Build history of the part. All positions in model axes, mm. A direction names the side the tool comes from. Round coordinates to 2 decimals unless told otherwise and drop trailing zeros. One line per question, with ' | ' between items.
Autodesk Inventor part; units mm, degrees
ref_plane "Work Plane1" through (-1.711, 0.0003, 0) normal (0, 1, 0) x (1, 0, 0)
ref_plane "Work Plane2" through (0.1135, 0.0003, 76.2) normal (0, 0, -1) x (-1, 0, 0)
ref_plane "YZ Plane" through (0, 0, 0) normal (1, 0, 0) x (0, 1, 0)
sketch "Sketch1" plane through (0, 0, 0) normal (0, 0, 1) x (1, 0, 0)
  line L0 (1.9552, -3.1747) -> (-1.711, -3.1747)
  line L1 (-1.711, -3.1747) -> (-3.5441, 0.0003)
  line L2 (-3.5441, 0.0003) -> (-1.711, 3.1753)
  line L3 (-1.711, 3.1753) -> (1.9552, 3.1753)
  line L4 (1.9552, 3.1753) -> (3.7883, 0.0003)
  line L5 (3.7883, 0.0003) -> (1.9552, -3.1747)
  point P0 (0.1221, 0.0003)
  dimension "d0" = 6.35
extrude "Extrusion1" add sketch "Sketch1" along normal blind 152.4
ref_plane "Work Plane1" through (-1.711, 0.0003, 0) normal (0, 1, 0) x (1, 0, 0)
sketch "Sketch3" plane through (-1.711, 0.0003, 0) normal (0, 1, 0) x (1, 0, 0)
  line L0 (-1.3251, 0) -> (4.9741, 0)
  line L1 (5.4821, -0.508) -> (5.4821, -151.892)
  line L2 (-1.8331, -151.892) -> (-1.8331, -0.508)
  line L3 (-1.8331, -0.508) -> (-1.3251, 0)
  line L4 (4.9741, 0) -> (5.4821, -0.508)
  line L5 (-1.8331, 0) -> (-1.8331, -152.4)
  line L6 (3.6662, 0) -> (5.4993, 0)
  line L7 (1.8245, 0) -> (1.8245, -152.4)
  line L8 (0, -152.4) -> (-1.8331, -152.4)
  line L9 (5.4993, -152.4) -> (3.6662, -152.4)
  line L10 (3.6662, -152.4) -> (0, -152.4)
  line L11 (-1.3251, -152.4) -> (-1.8331, -151.892)
  line L12 (4.9741, -152.4) -> (5.4821, -151.892)
  point P0 (-1.8331, 0)
  point P1 (5.4821, 0)
  point P2 (5.4821, -152.4)
  dimension "d5" = 0.508
  dimension "d6" = 0.508
  dimension "d7" = 0.508
  dimension "d8" = 0.508
  dimension "d16" = 0
  dimension "d46" = 0.508
  dimension "d47" = 0.508
  dimension "d48" = 0.508
  dimension "d49" = 0.508
revolve "Revolution1" cut sketch "Sketch3" angle 360 about axis through (0.1135, 0.0003, 0) along (0, 0, 1) keep common part contours L0 L4 L1 L12 L9 L10 L7
sketch "Sketch6" plane through (0.1135, 0.0003, 0) normal (0, 0, -1) x (-1, 0, 0)
  circle A0 centre (0, 0) radius 3.1496
hole "Hole3" at (0.1135, 0.0003, 0) direction (0, 0, 1) diameter 3.302 depth 12.7 tip angle 118
sketch "Sketch7" plane through (0, 0, 152.4) normal (0, 0, 1) x (1, 0, 0)
  point P0 (0, 0)
hole "Hole4" at (0, 0, 152.4) direction (0, 0, -1) diameter 3.302 depth 12.7 tip angle 118
ref_plane "Work Plane2" through (0.1135, 0.0003, 76.2) normal (0, 0, -1) x (-1, 0, 0)
properties part number "6 inch Standoff" material "Steel"
(1) Wall check: line 1 (X direction, y = 0, z = 146); line 2 (Y direction, x = 0, z = 148.75); line 3 (Y direction, x = 3.25, z = 52.5). Give the ranges that are in metal, low to high. Write a range as from..to.
Calculated:
line 1: -3.54..-1.65, 1.65..3.77 | line 2: -3.17..-1.65, 1.65..3.18 | line 3: -0.93..0.93
(2) Mould opens along X. For faces 4 (the conical face through (-0.3, 0.1, 138.9)), 5 (the flat face through (2.88, -1.57, 75.13)), 6 (the flat face through (0, 3.175, 75)), 7 (the conical face through (-0.14, 0.13, 13.52)) say: pulls with the +X half, pulls with the -X half, needs draft (parallel to the pull), parting line crosses it, or undercut.
Calculated:
face 4: undercut | face 5: pulls with the +X half | face 6: needs draft | face 7: undercut
(3) Drop flat-ended pins along their axis: pin 1 (3 mm diameter, centred on x = 0.11, y = 0, fed in from +Z); pin 2 (2.5 mm diameter, centred on x = 0, y = 0, fed in from +Z). Give the stop position or say it passes through.
Calculated:
pin 1: z = 139.68 | pin 2: z = 139.46
(4) 3-axis set-ups, long thin cutter, end or side, ignore diameter. For faces 1 (the flat face through (-2.617, -1.606, 75.133)), 2 (the cylindrical face through (1.725, -0.358, 6.439)), 3 (the cylindrical face through (0.632, -1.525, 145.961)): which of +Z, -Z, +X, -X, +Y, -Y reach the whole face in a straight line?
Calculated:
face 1: +Z, -Z, -X, -Y | face 2: -Z | face 3: +Z
